Design review of the part built by this model. Coordinates are the model's own, in mm. Face numbers are marked on the shaded views. A direction names the side the tool comes from. Give positions to 0.01 mm unless a question says otherwise; leave off trailing zeros. Write each loop counter-clockwise with the first axis right and the second up, starting at its lowest first coordinate (ties: lowest second). Pieces come first, ordered by that corner, then holes. Notation, with made-up numbers: (86.25, 66) -> (100.25, 66) arc R17 ccw to (100.25, 87) -> close; hole circle Ø9 at (-16, 56). An arc over 180 degrees is marked (long way). Return JSON: item names as keys, results as strings. Group by question number.
Autodesk Inventor part; units mm, degrees
ref_plane "YZ Plane" through (0, 0, 0) normal (1, 0, 0) x (0, 1, 0)
ref_plane "XZ Plane" through (0, 0, 0) normal (0, 1, 0) x (-1, 0, 0)
ref_plane "XY Plane" through (0, 0, 0) normal (0, 0, 1) x (1, 0, 0)
sketch "Sketch1" plane through (0, 0, 0) normal (0, 0, 1) x (1, 0, 0)
  line L0 (0, 0) -> (42.4, 0)
  line L1 (42.4, 0) -> (42.4, 24)
  line L2 (42.4, 24) -> (0, 24)
  line L3 (0, 24) -> (0, 0)
  circle A0 centre (9.2, 20) radius 2.1
  circle A1 centre (33.2, 20) radius 2.1
  circle A2 centre (33.2, 4) radius 2.1
  circle A3 centre (9.2, 4) radius 2.1
  dimension "d0" = 24
  dimension "d1" = 42.4
  dimension "d2" = 4.2
  dimension "d3" = 9.2
  dimension "d4" = 9.2
  dimension "d5" = 9.2
  dimension "d6" = 9.2
  dimension "d7" = 4
  dimension "d8" = 4
  dimension "d9" = 4
  dimension "d10" = 4
extrude "Extrusion1" add sketch "Sketch1" along normal blind 13.5
sketch "Sketch2" plane through (0, 0, 0) normal (0, -1, 0) x (1, 0, 0)
  line L0 (42.4, 13.5) -> (0, 13.5)
  line L1 (0, 0) -> (0, 13.5)
  circle A0 centre (21.2, 15) radius 7.5
  dimension "d13" = 15
  dimension "d14" = 21.2
  dimension "d15" = 1.5
extrude "Extrusion2" cut sketch "Sketch2" against normal through all
fillet "Fillet1" radius 3 3 edges at (42.4, 0, 6.75) (0, 0, 6.75) (21.2, 0, 0)
sketch "Sketch3" plane through (0, 0, 0) normal (0, 0, -1) x (-1, 0, 0)
  arc A0 (-31.3534, 3) -> (-35.0466, 3) centre (-33.2, 4) ccw
  arc A1 (-7.3534, 3) -> (-11.0466, 3) centre (-9.2, 4) ccw
  circle A2 centre (-33.2, 20) radius 2.1
  circle A3 centre (-9.2, 20) radius 2.1
  circle A4 centre (-33.2, 20) radius 4.25
  circle A5 centre (-9.2, 20) radius 4.25
  circle A6 centre (-9.2, 4) radius 4.25
  circle A7 centre (-33.2, 4) radius 4.25
  point P0 (0, 0)
  dimension "d20" = 8.5
extrude "Extrusion3" cut sketch "Sketch3" against normal blind 4
sketch "Sketch4" plane through (21.2, 0, 15) normal (0, -1, 0) x (1, 0, 0)
  line L0 (-26.3081, 1.9971) -> (24.247, 1.9971)
  line L1 (24.247, 1.9971) -> (24.247, -18.7305)
  line L2 (24.247, -18.7305) -> (-26.3081, -18.7305)
  line L3 (-26.3081, -18.7305) -> (-26.3081, 1.9971)
  point P0 (-21.2, -15)
extrude "Extrusion4" cut sketch "Sketch4" against normal blind 12.3
fillet "Fillet3" radius 3 2 edges at (42.4, 18.15, 0) (0, 18.15, 0)
fillet "Fillet4" radius 1 7 edges at (41.5213, 24, 0.8787) (37.0181, 24, 0) (42.4, 24, 8.25) (21.2, 24, 0) (0.8787, 24, 0.8787) (0, 24, 8.25) (5.3819, 24, 0)
properties part number "Z move clamp small"
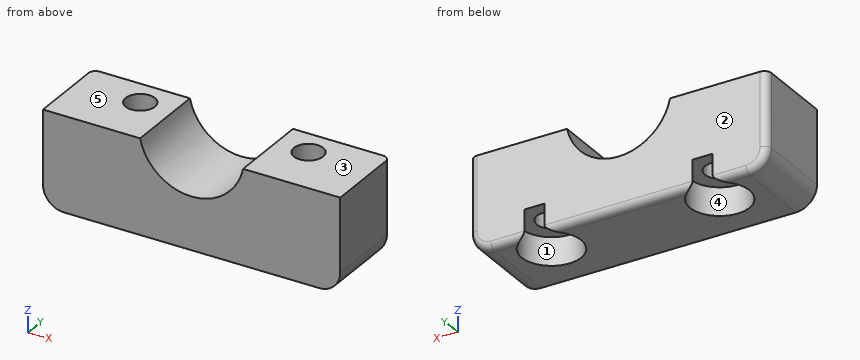
Q1. Insertion check: pin 1 (5 mm diameter, centred on x = 9.2, y = 20, fed in from -Z); pin 2 (2 mm diameter, centred on x = 4.5, y = 18, fed in from -Z). Each pin has a flat end and moves straight along its axis. Give the tip position at first contact, or say it passes through.
Q2. For L1, parallel to X at y = 18.5, z = 2.25; L2, parallel to X at y = 21.75, z = 10.75; L3, parallel to Y at x = 9.2, z = 11, list the stretches that pass through material, from the lowest coordinate up. Write a range as from..to.
Q3. Take a section at D-D, the plane y = 14.5. Give the boundary of the cut face in (x, z), plus the area to 3 significant figures.
Q4. Take a section at A-A, the plane x = 33.2. Give the boundary of the cut face in (y, z), plus the area to 4 significant figures.
Q5. Take a section at C-C, the plane z = 9.5. Give the boundary of the cut face in (x, y), plus the area to 3 significant figures.
Q6. Take a section at B-B, the plane y = 20. Give the boundary of the cut face in (x, z), plus the area to 3 significant figures.
Q7. Mouldability with a two-part tool opening along Y and no side actions: class the marked faces 1, 2 and 3 as +Y half, -Y half, draft (parallel to the pull), parting line (faces both ways), or undercut.
Q8. Tool access review of the marked faces 4 and 5: name each direction out of +Z, -Z, +X, -X, +Y, -Y from which nothing blocks a thin tool from reaching the whole face with its end or side.
Final values:
{
 "1": {"pin 1": "stops at z = 4", "pin 2": "stops at z = 0"},
 "2": {"L1": "x = 0.1..5.22, 13.18..29.22, 37.18..42.3", "L2": "x = 0..8.04, 10.36..15.02, 27.38..32.04, 34.36..42.4", "L3": "y = 12.3..17.9, 22.1..24"},
 "3": {"outline": "(0, 3) arc R3 ccw to (3, 0) -> (39.4, 0) arc R3 ccw to (42.4, 3) -> (42.4, 13.5) -> (28.55, 13.5) arc R7.5 cw to (13.85, 13.5) -> (0, 13.5) -> close", "area": "503 mm²"},
 "4": {"outline": "(12.3, 0) -> (15.75, 0) -> (15.75, 4) -> (17.9, 4) -> (17.9, 13.5) -> (12.3, 13.5) -> close; (22.1, 4) -> (24, 4) -> (24, 13.5) -> (22.1, 13.5) -> close", "area": "85.05 mm²"},
 "5": {"outline": "(0, 12.3) -> (16.1, 12.3) -> (16.1, 24) -> (1, 24) arc R1 ccw to (0, 23) -> close; (26.3, 12.3) -> (42.4, 12.3) -> (42.4, 23) arc R1 ccw to (41.4, 24) -> (26.3, 24) -> close; hole circle Ø4.2 at (9.2, 20); hole circle Ø4.2 at (33.2, 20)", "area": "349 mm²"},
 "6": {"outline": "(0, 3) arc R3 ccw to (3, 0) -> (4.95, 0) -> (4.95, 4) -> (7.1, 4) -> (7.1, 13.5) -> (0, 13.5) -> close; (11.3, 4) -> (13.45, 4) -> (13.45, 0) -> (28.95, 0) -> (28.95, 4) -> (31.1, 4) -> (31.1, 13.5) -> (28.55, 13.5) arc R7.5 cw to (13.85, 13.5) -> (11.3, 13.5) -> close; (35.3, 4) -> (37.45, 4) -> (37.45, 0) -> (39.4, 0) arc R3 ccw to (42.4, 3) -> (42.4, 13.5) -> (35.3, 13.5) -> close", "area": "355 mm²"},
 "7": {"face 1": "undercut", "face 2": "+Y half", "face 3": "draft"},
 "8": {"face 4": "-Z", "face 5": "+Z, +X, -X, +Y, -Y"}
}
